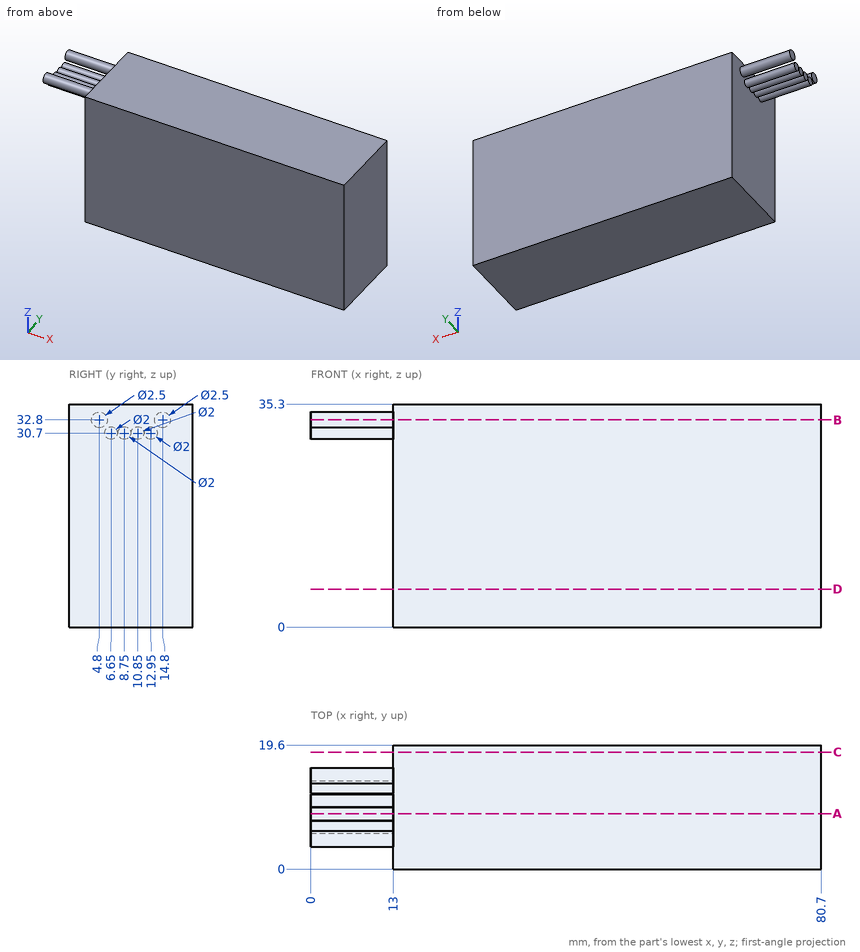
Drawing for the job (mm, zero at the part's lowest x, y, z). Give positions to 0.01 mm unless a question says otherwise; leave off trailing zeros. Loops run counter-clockwise (first coordinate to the right, second up) from the corner with the lowest first, then second, coordinate; pieces in that order, holes last. Notation, with made-up numbers: M -0.5,63 L 18.5,63 A30 cw 18.5,102 Z; hole C -4,28.25 d6. An arc over 180 degrees is marked long. Use one line per item in the form item = value.
Item 1: Slice it at A-A (y = 8.75). List the corners of the cut face in (x, z), plus the area to 3 significant figures.
Determined:
outline = M 0,29.7 L 13,29.7 L 13,0 L 80.7,0 L 80.7,35.3 L 13,35.3 L 13,31.7 L 0,31.7 Z
area = 2,420 mm2
Item 2: Slice it at C-C (y = 18.5). List the corners of the cut face in (x, z), plus the area to 3 significant figures.
Determined:
outline = M 13,0 L 80.7,0 L 80.7,35.3 L 13,35.3 Z
area = 2,390 mm2
Item 3: Slice it at B-B (z = 32.8). List the corners of the cut face in (x, y).
Determined:
outline = M 0,3.55 L 13,3.55 L 13,0 L 80.7,0 L 80.7,19.6 L 13,19.6 L 13,16.05 L 0,16.05 L 0,13.55 L 13,13.55 L 13,6.05 L 0,6.05 Z
Item 4: Drill centre line: probe 1 along X at (y, z) = (11.75, 11.5). Where is it in solid material? Low to high. Write a range as from..to.
Determined:
probe_1 = 13..80.7
Item 5: Flat gauge pins, fed straight in: pin 1 (6 mm diameter, centred on x = 8.5, y = 9.5, fed in from +Z); pin 2 (6 mm diameter, centred on y = 9.5, z = 18.5, fed in from -X). Where does each tip first touch, or does it go through?
Determined:
pin_1 = 31.7
pin_2 = 13
Item 6: Slice it at D-D (z = 6). List the corners of the cut face in (x, y).
Determined:
outline = M 13,0 L 80.7,0 L 80.7,19.6 L 13,19.6 Z
